from build123d import *

# Parameters (mm, degrees)
SKETCH1_W           = 119
SKETCH1_H           = 90
SKETCH1_R           = 6.25
SKETCH1_W_2         = 7.5
SKETCH1_H_2         = 7.5
BOSS_EXTRUDE1_DEPTH = 5
SKETCH1_3_W         = 4.5
SKETCH1_3_H         = 4.5
SKETCH1_3_W_2       = 2.5
SKETCH1_3_H_2       = 2.5
BOSS_EXTRUDE2_DEPTH = 13


with BuildPart() as part:
    # Sketch1 → Boss-Extrude1 (new body)
    with BuildSketch(Plane.XY):
        with Locations((34.214905029, -83.582846692)):
            Rectangle(SKETCH1_W, SKETCH1_H)
        with Locations((33.949905029, -113.682846692)):
            Circle(SKETCH1_R, mode=Mode.SUBTRACT)
        with Locations((54.399905029, -107.282846692)):
            Rectangle(SKETCH1_W_2, SKETCH1_H_2, mode=Mode.SUBTRACT)
    extrude(amount=BOSS_EXTRUDE1_DEPTH)

    # Sketch1_3 → Boss-Extrude2 (add)
    with BuildSketch(Plane.XY):
        with Locations((78.199905029, -121.282846692)):
            Rectangle(SKETCH1_3_W, SKETCH1_3_H)
        with Locations((-11.560094971, -43.782846692)):
            Rectangle(SKETCH1_3_W_2, SKETCH1_3_H_2)
        with Locations((79.199905029, -43.782846692)):
            Rectangle(SKETCH1_3_W_2, SKETCH1_3_H_2)
    extrude(amount=BOSS_EXTRUDE2_DEPTH)


solid = part.part
Read the model definition and answer for the solid it produces. Units are mm, in the model's axes. A direction names the side the tool comes from. Round coordinates to 2 decimals unless told otherwise and drop trailing zeros. Loops run counter-clockwise (first coordinate to the right, second up) from the corner with the lowest first, then second, coordinate; pieces in that order, holes last.
Q1. Section D-D on y = -93 is taken. Write down the section's boundary in (x, z).
Q2. Each of these flat-tipped pins is pushed along its axis until it touches: pin 1 (1.2 mm diameter, centred on x = 79.5, z = 10, fed in from -Y); pin 2 (3 mm diameter, centred on x = 41.5, y = -57.5, fed in from +Z); pin 3 (3 mm diameter, centred on y = -43.5, z = 7, fed in from +X); pin 4 (5 mm diameter, centred on x = 7, z = 8.5, fed in from +Y). Where does it stop, or does it pass through?
Q3. Section B-B on z = 7.5 is taken. Write down the section's boundary in (x, y), and give its area (4 significant figures).
Q4. Which of the six approach directions +Z, -Z, +X, -X, +Y, -Y give full straight-line access (tool end or side, diameter ignored) to faces 5 (the face through (-12, -45.033, 9)), 6 (the face through (80.45, -44, 9)), 7 (the face through (75.95, -121, 9)), 8 (the face through (54, -103.533, 2))?
Q5. Section C-C on x = 55 is taken. Write down the section's boundary in (y, z).
Q6. Determine the mould class of faces 1 (the face through (79, -42.533, 9)), 2 (the face through (77.95, -44, 9)), 3 (the face through (-12.81, -44, 9)), 4 (the face through (32.595, -119.784, 2.465)) for opening direction X: released by +X, released by -X, zero draft, split by the parting line, or undercut.
Q7. Consider probe 1 along X at (y, z) = (-43.5, 11); probe 2 along Z at (x, y) = (81, -123.5); probe 3 along Y at (x, z) = (55, 1.5). Determine where each line is inside the solid, lowest interval first.
Q8. Section A-A on x = 37 is taken. Write down the section's boundary in (y, z).
Output:
1. outline: (-25.29, 0) - (93.71, 0) - (93.71, 5) - (-25.29, 5) - close
2. pin 1: stops at y = -123.53
2. pin 2: stops at z = 5
2. pin 3: stops at x = 80.45
2. pin 4: passes through
3. outline: (-12.81, -45.03) - (-10.31, -45.03) - (-10.31, -42.53) - (-12.81, -42.53) - close; (75.95, -123.53) - (80.45, -123.53) - (80.45, -119.03) - (75.95, -119.03) - close; (77.95, -45.03) - (80.45, -45.03) - (80.45, -42.53) - (77.95, -42.53) - close
3. area: 32.75 mm2
4. face 5: +Z, +X, -X, -Y
4. face 6: +Z, +X, +Y, -Y
4. face 7: +Z, -X, +Y, -Y
4. face 8: +Z, -Z
5. outline: (-128.58, 0) - (-111.03, 0) - (-111.03, 5) - (-128.58, 5) - close; (-103.53, 0) - (-38.58, 0) - (-38.58, 5) - (-103.53, 5) - close
6. face 1: zero draft
6. face 2: undercut
6. face 3: released by -X
6. face 4: undercut
7. probe 1: x = -12.81 to -10.31, 77.95 to 80.45
7. probe 2: z = 0 to 5
7. probe 3: y = -128.58 to -111.03, -103.53 to -38.58
8. outline: (-128.58, 0) - (-119.14, 0) - (-119.14, 5) - (-128.58, 5) - close; (-108.23, 0) - (-38.58, 0) - (-38.58, 5) - (-108.23, 5) - close
